For this review, take the finished solid that the model builds, in its own axes (mm). Face numbers are marked on the shaded views. A direction names the side the tool comes from. Coordinates: 2 decimals unless noted, no trailing zeros. Loops run counter-clockwise (first coordinate to the right, second up) from the corner with the lowest first, then second, coordinate; pieces in that order, holes last. Notation, with made-up numbers: M -12.75,75.5 L 27.25,75.5 A20 cw 27.25,88.5 Z; hole C 55.25,15 d3. An arc over 180 degrees is marked long. Use one line per item in the form item = value.
```python
from build123d import *

# Parameters (mm, degrees)
SKETCH1_W           = 36
SKETCH1_H           = 55
BOSS_EXTRUDE1_DEPTH = 3
SKETCH2_W           = 36
SKETCH2_H           = 55
SKETCH2_W_2         = 30.4
SKETCH2_H_2         = 49.3
BOSS_EXTRUDE2_DEPTH = 7
SKETCH3_W           = 30.4
SKETCH3_H           = 31
CUT_EXTRUDE1_DEPTH  = 1.5


with BuildPart() as part:
    # Sketch1 → Boss-Extrude1 (new body)
    with BuildSketch(Plane(origin=(0, 0, 0), x_dir=(1, 0, 0), z_dir=(0, 1, 0))):
        with Locations((18, 27.5)):
            Rectangle(SKETCH1_W, SKETCH1_H)
    extrude(amount=BOSS_EXTRUDE1_DEPTH)

    # Sketch2 → Boss-Extrude2 (add)
    with BuildSketch(Plane(origin=(0, 3, 0), x_dir=(1, 0, 0), z_dir=(0, 1, 0))):
        with Locations((18, 27.5)):
            Rectangle(SKETCH2_W, SKETCH2_H)
        with Locations((18, 27.5)):
            Rectangle(SKETCH2_W_2, SKETCH2_H_2, mode=Mode.SUBTRACT)
    extrude(amount=BOSS_EXTRUDE2_DEPTH)

    # Sketch3 → Cut-Extrude1 (cut)
    with BuildSketch(Plane(origin=(0, 3, 0), x_dir=(1, 0, 0), z_dir=(0, 1, 0))):
        with Locations((18, 36.65)):
            Rectangle(SKETCH3_W, SKETCH3_H)
    extrude(amount=-CUT_EXTRUDE1_DEPTH, mode=Mode.SUBTRACT)


solid = part.part
```
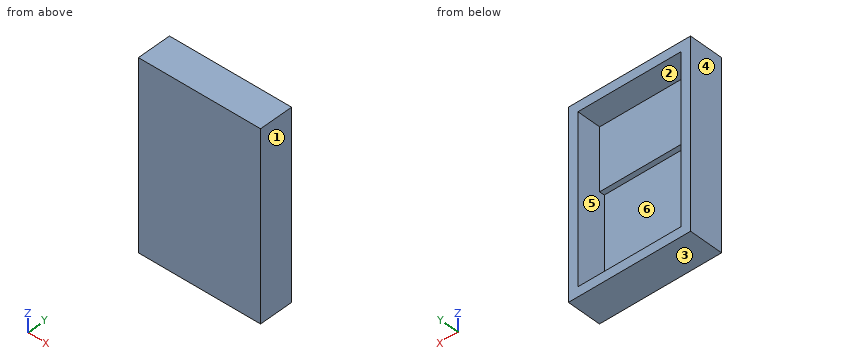
1. Consider section A-A on y = 6.5. Write out the cut boundary in (x, z).
Computed values:
outline = M 0,-55 L 36,-55 L 36,0 L 0,0 Z; hole M 2.8,-52.15 L 33.2,-52.15 L 33.2,-2.85 L 2.8,-2.85 Z
2. For pin 1 Ø1.5 at (x, z) = (17, -8) entering from +Y; pin 2 Ø6 at (x, y) = (9, 7.5) entering from +Z; pin 3 Ø5 at (x, z) = (7, -29) entering from +Y, all flat-tipped, find the tip position at first contact; note any pin that passes through.
Computed values:
pin_1 = 3
pin_2 = 0
pin_3 = 1.5
3. Consider section D-D on z = -10.5. Write out the cut boundary in (x, y), plus the area to 3 significant figures.
Computed values:
outline = M 0,0 L 36,0 L 36,10 L 33.2,10 L 33.2,3 L 2.8,3 L 2.8,10 L 0,10 Z
area = 147 mm2
4. Consider section B-B on z = -37.5. Write out the cut boundary in (x, y), plus the area to 3 significant figures.
Computed values:
outline = M 0,0 L 36,0 L 36,10 L 33.2,10 L 33.2,1.5 L 2.8,1.5 L 2.8,10 L 0,10 Z
area = 102 mm2
5. Consider section C-C on x = 23.5. Write out the cut boundary in (y, z).
Computed values:
outline = M 0,-55 L 10,-55 L 10,-52.15 L 1.5,-52.15 L 1.5,-21.15 L 3,-21.15 L 3,-2.85 L 10,-2.85 L 10,0 L 0,0 Z
6. Draft analysis for pull direction Z (two halves, no side actions). For the marked faces 3, 4, 5 and 6, state which applies: +Z half, -Z half, draft (parallel to the pull), parting line (faces both ways), or undercut.
Computed values:
face_3 = -Z half
face_4 = draft
face_5 = undercut
face_6 = undercut
7. Wall thickness on line 1 along X through (y, z) = (8.5, -25.5); line 2 along Z through (x, y) = (19.5, 7.75); line 3 along Y through (x, z) = (24.5, -32): over which ranges is each line inside the solid? List them lowest first. Write a range as from..to.
Computed values:
line_1 = 0..2.8, 33.2..36
line_2 = -55..-52.15, -2.85..0
line_3 = 0..1.5
8. Tool access review of the marked faces 1 and 2: name each direction out of +Z, -Z, +X, -X, +Y, -Y from which nothing blocks a thin tool from reaching the whole face with its end or side.
Computed values:
face_1 = +Z, -Z, +X, +Y, -Y
face_2 = +Y
